The listing builds one solid part. Answer for the finished solid, in the listing's coordinates (mm). A direction names the side the tool comes from. Coordinates: 2 decimals unless noted, no trailing zeros. Loops run counter-clockwise (first coordinate to the right, second up) from the corner with the lowest first, then second, coordinate; pieces in that order, holes last. Notation, with made-up numbers: (4.25, 4.5) - (48.25, 4.5) arc R22 ccw to (48.25, 24.5) - close; hole circle Ø4 at (27, -2). An arc over 180 degrees is marked (long way). Put each result on its own line as item: value.
```python
from build123d import *

# Parameters (mm, degrees)
F2_R = 1.27
F3_R = 1.27


with BuildPart() as f1:
    # F0 (on Front) → F1 (revolve)
    with BuildSketch(Plane.XZ):
        Polygon((-28.575, 0), (0, 0), (0, 101.6), (-11.43, 101.6), (-27.94, 17.78), (-29.21, 14.605), (-31.75, 14.605), (-31.75, 3.175), (-28.575, 3.175), align=None)
    revolve(axis=Axis((0, 0, 50.8), (0, 0, -1)))

    # F2
    f2_edges = [f1.edges().sort_by_distance(p)[0] for p in [
        (29.21, 0, 14.605),
    ]]
    fillet(f2_edges, radius=F2_R)

    # F3
    f3_edges = [f1.edges().sort_by_distance(p)[0] for p in [
        (31.75, 0, 14.605),
    ]]
    fillet(f3_edges, radius=F3_R)


solid = f1.part
```
1) Straight lines are drawn through the part: L1, parallel to Z at x = -26.5, y = 14.5 (3 decimals); L2, parallel to Y at x = -12.5, z = 63; L3, parallel to Y at x = 15, z = 66.5. For each, find the intervals that lie inside material, in ascending order. Write a range as [from, to].
Found:
L1: z = [3.175, 14.605]
L2: y = [-14.35, 14.35]
L3: y = [-10.56, 10.56]
2) For faces 1 (the face through (-13.7, -27, 14.605)), 2 (the face through (28.4, 4.9, 3.175)), 3 (the face through (0, 0, 101.6)), determine the directions among +Z, -Z, +X, -X, +Y, -Y from which every point of the face is accessible in a straight line to the end or side of a thin tool.
Found:
face 1: +Z
face 2: -Z
face 3: +Z, +X, -X, +Y, -Y
3) Each of these flat-tipped pins is pushed along its axis until it touches: pin 1 (2 mm diameter, centred on y = 9, z = 39, fed in from -X); pin 2 (12 mm diameter, centred on y = 4.5, z = 89, fed in from +X); pin 3 (6 mm diameter, centred on y = 2, z = 46, fed in from -X). Where does it stop, or does it pass through?
Found:
pin 1: stops at x = -22.43
pin 2: stops at x = 14.86
pin 3: stops at x = -22.92
4) The part is cut by section C-C (z = 56.5). Give the vertices of the cut face in (x, y), and give its area (3 significant figures).
Found:
outline: circle Ø40.63 at (0, 0)
area: 1,300 mm^2
5) The part is cut by section A-A (y = 0). Give the vertices of the cut face in (x, z) (3 decimals).
Found:
outline: (-31.75, 3.175) - (-28.575, 3.175) - (-28.575, 0) - (28.575, 0) - (28.575, 3.175) - (31.75, 3.175) - (31.75, 13.335) arc R1.27 ccw to (30.48, 14.605) - (30.07, 14.605) arc R1.27 cw to (28.891, 15.403) - (27.94, 17.78) - (11.43, 101.6) - (-11.43, 101.6) - (-27.94, 17.78) - (-28.891, 15.403) arc R1.27 cw to (-30.07, 14.605) - (-30.48, 14.605) arc R1.27 ccw to (-31.75, 13.335) - close
6) The part is cut by section D-D (z = 85). Give the vertices of the cut face in (x, y).
Found:
outline: circle Ø29.4 at (0, 0)
